from build123d import *

# Parameters (mm, degrees)
F0_W     = 8
F0_H     = 6
F0_H_2   = 5.6374937892
F0_W_2   = 4
F0_H_3   = 23
F1_DEPTH = 7
F2_D     = 2
F3_D     = 5.75


with BuildPart() as f1:
    # F0 (on Top) → F1 (new body)
    with BuildSketch(Plane.XY):
        Polygon((10.5, -45), (22.5, -45), (22.5, -10.6539065018), (22.5, 17.153987661), (0, 45), (-14.5, 45), (-14.5, 39), (-14.5, 16), (-14.5, 10.3625062108), (-22.5, 10.3625062108), (-22.5, -42.25), (-10.5080957781, -42.25), (-10.6281967604, -1.0001864958), (10.3717142302, -0.9390441602), align=None)
        Polygon((0, 45), (22.5, 17.153987661), (22.5, 45), align=None)
        Polygon((-30.5, 39), (-30.5, 45), (-55.0723059862, 45), (-55.0723059862, 10.3625062108), (-30.5, 10.3625062108), (-30.5, 16), align=None)
        with Locations((-26.5, 42)):
            Rectangle(F0_W, F0_H)
        Polygon((-14.5, 39), (-14.5, 45), (-22.5, 45), (-22.5, 39), (-18.5, 39), align=None)
        Polygon((-22.5, 16), (-22.5, 10.3625062108), (-14.5, 10.3625062108), (-14.5, 16), (-18.5, 16), align=None)
        with Locations((-26.5, 13.1812531054)):
            Rectangle(F0_W, F0_H_2)
        Polygon((22.5, 17.153987661), (22.5, -10.6539065018), (60.7781559229, -10.6539065018), (60.7781559229, 45), (22.5, 45), align=None)
        Polygon((0, 45), (22.5, 45), (60.7781559229, 45), (60.6384575367, 56.7700602114), (-55.0723059862, 56.7700602114), (-55.0723059862, 45), (-30.5, 45), (-22.5, 45), (-14.5, 45), align=None)
        with Locations((-16.5, 27.5)):
            Rectangle(F0_W_2, F0_H_3)
    extrude(amount=F1_DEPTH)

    # F2 (through all)
    with Locations(Plane(origin=(0, 0, 0), x_dir=(1, 0, 0), z_dir=(0, 0, -1))):
        with Locations((-17.0669870824, 5), (-17.7734121563, 37), (17.7265878437, 39), (17.9330129176, 7)):
            Hole(F2_D / 2)

    # F3 (through all)
    with Locations(Plane(origin=(0, 0, 0), x_dir=(1, 0, 0), z_dir=(0, 0, -1))):
        with Locations((-10.5364832571, 32.5000529818), (10.4634277335, 32.4389106462)):
            Hole(F3_D / 2)


solid = f1.part
Here's how the part is built. I have some questions about the finished solid (model axes, mm). A direction names the side the tool comes from. Give positions to 0.01 mm unless a question says otherwise; leave off trailing zeros. Loops run counter-clockwise (first coordinate to the right, second up) from the corner with the lowest first, then second, coordinate; pieces in that order, holes last. Notation, with made-up numbers: (8, 50.25) -> (56, 50.25) arc R18 ccw to (56, 61.25) -> close; hole circle Ø3 at (46, 19). An arc over 180 degrees is marked (long way). Answer as a JSON object with one key per item and string values. Group by question number.
Item 1: On a 3-axis mill with a long thin cutter (end or side, diameter ignored), from which of +Z, -Z, +X, -X, +Y, -Y can I reach the whole of each face in a straight line? I mean faces 1 (the flat face through (16, -45, 3)), 2 (the flat face through (-39, 10.363, 3)), 3 (the flat face through (41, -10.654, 3)), 4 (the flat face through (-24, 16, 3)), 5 (the flat face through (-55.072, 34, 3)). Say none if no direction works.
Item 2: Imagine slicing it at A-A on z = 3. Give the number of separate pieces and of enclosed holes in the cut face, then the cut area to 3 significant figures.
Item 3: Imagine slicing it at B-B on y = 33. Write out the boundary of the cut face in (x, z).
Item 4: Will these pins go through, and if not, where does the flat tip stop? pin 1 (2 mm diameter, centred on x = -24, z = 2.5, fed in from -Y); pin 2 (4 mm diameter, centred on x = 39, z = 1.5, fed in from -Y); pin 3 (1.6 mm diameter, centred on x = -17.07, y = -5, fed in from -Z); pin 4 (3.5 mm diameter, centred on y = -13, z = 3.5, fed in from -X).
Item 5: Thinking about a two-plate mould opening in Y: for faces 6 (the flat face through (-18.5, 27, 3)), 7 (the flat face through (60.778, 17, 3)), 8 (the cylindrical face through (13.338, -32.494, 3.549)), 9 (the flat face through (-17, -42.25, 3)), which applies, pulls with the +Y half, pulls with the -Y half, needs draft (parallel to the pull), parting line crosses it, or undercut?
Item 6: Imagine slicing it at C-C on x = 35. Write out the boundary of the cut face in (y, z).
Item 7: I need wall thicknesses on L1, parallel to X at y = -5, z = 4; L2, parallel to X at y = -37, z = 2.5; L3, parallel to X at y = -9.5, z = 1.75. Which ranges of each line are inside material? Lowest first, please.
Item 8: Imagine slicing it at D-D on x = -48. Write out the boundary of the cut face in (y, z), then the cut area to 3 significant figures.
Answer list:
{
 "1": {"face 1": "+Z, -Z, +X, -X, -Y", "face 2": "+Z, -Z, -X, -Y", "face 3": "+Z, -Z, +X, -Y", "face 4": "+Z, -Z", "face 5": "+Z, -Z, -X, +Y, -Y"},
 "2": {"separate pieces": "1", "enclosed holes": "5", "area": "7,400 mm2"},
 "3": {"outline": "(-55.07, 0) -> (-30.5, 0) -> (-30.5, 7) -> (-55.07, 7) -> close; (-18.5, 0) -> (60.78, 0) -> (60.78, 7) -> (-18.5, 7) -> close"},
 "4": {"pin 1": "stops at y = 10.36", "pin 2": "stops at y = -10.65", "pin 3": "passes through", "pin 4": "stops at x = -22.5"},
 "5": {"face 6": "undercut", "face 7": "needs draft", "face 8": "undercut", "face 9": "pulls with the -Y half"},
 "6": {"outline": "(-10.65, 0) -> (56.77, 0) -> (56.77, 7) -> (-10.65, 7) -> close"},
 "7": {"L1": "x = -22.5 to -18.07, -16.07 to -10.62, 10.38 to 60.78", "L2": "x = -22.5 to -18.77, -16.77 to -10.52, 10.48 to 22.5", "L3": "x = -22.5 to -10.6, 10.4 to 60.78"},
 "8": {"outline": "(10.36, 0) -> (56.77, 0) -> (56.77, 7) -> (10.36, 7) -> close", "area": "325 mm2"}
}
